from build123d import *

# Parameters (mm, degrees)
BOSS_EXTRUDE1_DEPTH = 10
CUT_EXTRUDE1_DEPTH  = 21
BOSS_EXTRUDE2_REACH = 20.66
SKETCH3_R           = 3


with BuildPart() as part:
    # Sketch1 → Boss-Extrude1 (new body, symmetric)
    with BuildSketch(Plane.XY):
        Polygon((0, 0), (55, 0), (55, 10), (20, 10), (20, 32), (0, 32), align=None)
    extrude(amount=BOSS_EXTRUDE1_DEPTH, both=True)

    # Sketch2 → Cut-Extrude1 (cut, through all)
    with BuildSketch(Plane(origin=(20, 0, 0), x_dir=(0, 0, -1), z_dir=(1, 0, 0))):
        with BuildLine():
            Line((-1, 32), (1, 32))
            Line((1, 32), (1, 21.872983346))
            ThreePointArc((1, 21.872983346), (0, 14), (-1, 21.872983346))
            Line((-1, 21.872983346), (-1, 32))
        make_face()
    extrude(amount=-CUT_EXTRUDE1_DEPTH, mode=Mode.SUBTRACT)

    # Sketch3 → Boss-Extrude2 (add, up to next)
    with BuildSketch(Plane(origin=(0, 11.830127019, 6.830127019), x_dir=(-1, 0, 0), z_dir=(0, 0.866025404, 0.5)), mode=Mode.PRIVATE) as boss_extrude2_sk1:
        with BuildLine():
            Line((-47, 3.660254038), (-35, 3.660254038))
            Line((-35, 3.660254038), (-35, -4.339745962))
            ThreePointArc((-35, -4.339745962), (-41, -10.339745962), (-47, -4.339745962))
            Line((-47, -4.339745962), (-47, 3.660254038))
        make_face()
        with Locations(Location((-41, -4.339745962, 0), (0, 0, 90))):  # turned: the seam where the file's is
            Circle(SKETCH3_R, mode=Mode.SUBTRACT)
    boss_extrude2_tool1 = extrude(boss_extrude2_sk1.sketch, amount=-BOSS_EXTRUDE2_REACH, mode=Mode.PRIVATE) - part.part
    add(boss_extrude2_tool1.solids().sort_by_distance((41, 10.092195, 9.840313))[0])


solid = part.part
Verification items for the finished model (mm, model axes). A direction names the side the tool comes from. Coordinates: 2 decimals unless noted, no trailing zeros. Loops run counter-clockwise (first coordinate to the right, second up) from the corner with the lowest first, then second, coordinate; pieces in that order, holes last. Notation, with made-up numbers: M -7.5,82 L 13.5,82 A16 cw 13.5,108 Z; hole C 67,-15.5 d6. An arc over 180 degrees is marked long. One line per item, written item: value.
1. Set-up check for faces 5 (the flat face through (40.916, 11.895, 6.717)), 6 (the cylindrical face through (10, 14, 0)), 7 (the flat face through (10, 27, 1)): record each of +Z, -Z, +X, -X, +Y, -Y from which the full face is reachable in a straight line by a thin tool's end or side.
Answers follow:
face 5: +Z, +X, +Y
face 6: -X
face 7: +X, -X, +Y
2. Mould release check, pull along X, two halves, no side actions. Record for faces 1 (the flat face through (55, 5, 0)), 2 (the flat face through (21, 9, 10)), 3 (the flat face through (0, 13, 0)), 4 (the flat face through (41, 10, 1)): pulls with the +X half, pulls with the -X half, needs draft (parallel to the pull), parting line crosses it, or undercut.
Answers follow:
face 1: pulls with the +X half
face 2: needs draft
face 3: pulls with the -X half
face 4: undercut
3. Section check A-A on y = 18. Record the cut outline in (x, z).
Answers follow:
outline: M 0,-10 L 20,-10 L 20,-4 L 0,-4 Z; M 0,4 L 20,4 L 20,10 L 0,10 Z
4. Material ranges on line 1 along Z through (x, y) = (15, 30); line 2 along Z through (x, y) = (16, 18); line 3 along X through (y, z) = (14, 2), recorded low to high. Write a range as from..to.
Answers follow:
line 1: -10..-1, 1..10
line 2: -10..-4, 4..10
line 3: 0..20, 35.07..38.15, 43.85..46.93
5. Gauge pin test, flat ends, axial feed: P1, Ø4, axis at x = 18.5, z = 6, coming from the -Y side; P2, Ø10, axis at y = 23.5, z = -5, coming from the +X side; P3, Ø5, axis at y = 18, z = 0, coming from the -X side; P4, Ø3, axis at y = 15, z = -4, coming from the +X side. Record the tip position at first contact, or that the pin passes through.
Answers follow:
P1: y = 0
P2: x = 20
P3: x = 35.84
P4: x = 44.12
6. Section check B-B on z = -8.25. Record the cut outline in (x, y).
Answers follow:
outline: M 0,0 L 55,0 L 55,10 L 20,10 L 20,32 L 0,32 Z
7. Section check C-C on x = 49. Record the cut outline in (y, z), plus the area to 3 significant figures.
Answers follow:
outline: M 0,-10 L 10,-10 L 10,10 L 0,10 Z
area: 200 mm^2
8. Section check D-D on z = 8.25. Record the cut outline in (x, y).
Answers follow:
outline: M 0,0 L 55,0 L 55,10 L 47,10 L 47,11.01 L 35,11.01 L 35,10 L 20,10 L 20,32 L 0,32 Z
